Could you check a few things on this drawing? It's one solid part, dimensions in mm from its lowest x, y, z. A direction names the side the tool comes from. Coordinates: 2 decimals unless noted, no trailing zeros. Order: outer loops, then holes, each group sorted by start corner. A loop starts at its lowest first (then second) coordinate and runs counter-clockwise, first axis right, second up. Notation, with made-up numbers: (0, 53.5) -> (14, 53.5) arc R30 ccw to (14, 75.5) -> close; hole circle Ø5 at (-32, 24.25). An arc over 180 degrees is marked (long way). Use a Markdown table: item, result. Add a question column.
1. For the marked faces 1, 2 and 3, which set-ups out of +Z, -Z, +X, -X, +Y, -Y let a thin tool reach every point of the face, with its end or its side?
2. Suppose I cut it at A-A, the plane z = 8. List the corners of the cut face in (x, y) for me.
3. If I drill on line 1 along Z through (x, y) = (110, 14.5); line 2 along X through (y, z) = (2.75, 19); line 3 along X through (y, z) = (6.25, 17), over which ranges is the centre line in solid material (lowest first)? Write a range as from..to.
4. For pin 1 Ø5.5 at (y, z) = (10.5, 83.5) entering from +X; pin 2 Ø7 at (x, y) = (84.5, 11.5) entering from +Z; pin 3 Ø9 at (x, y) = (80.5, 8.5) entering from -Z, each with a flat end and sliding along its axis, tell me the tip position at first contact or that it passes through.
5. We'd pull the mould along X, two halves only. Please class the marked faces 4, 5, 6 and 7: pulls with the +X half, pulls with the -X half, needs draft (parallel to the pull), parting line crosses it, or undercut.
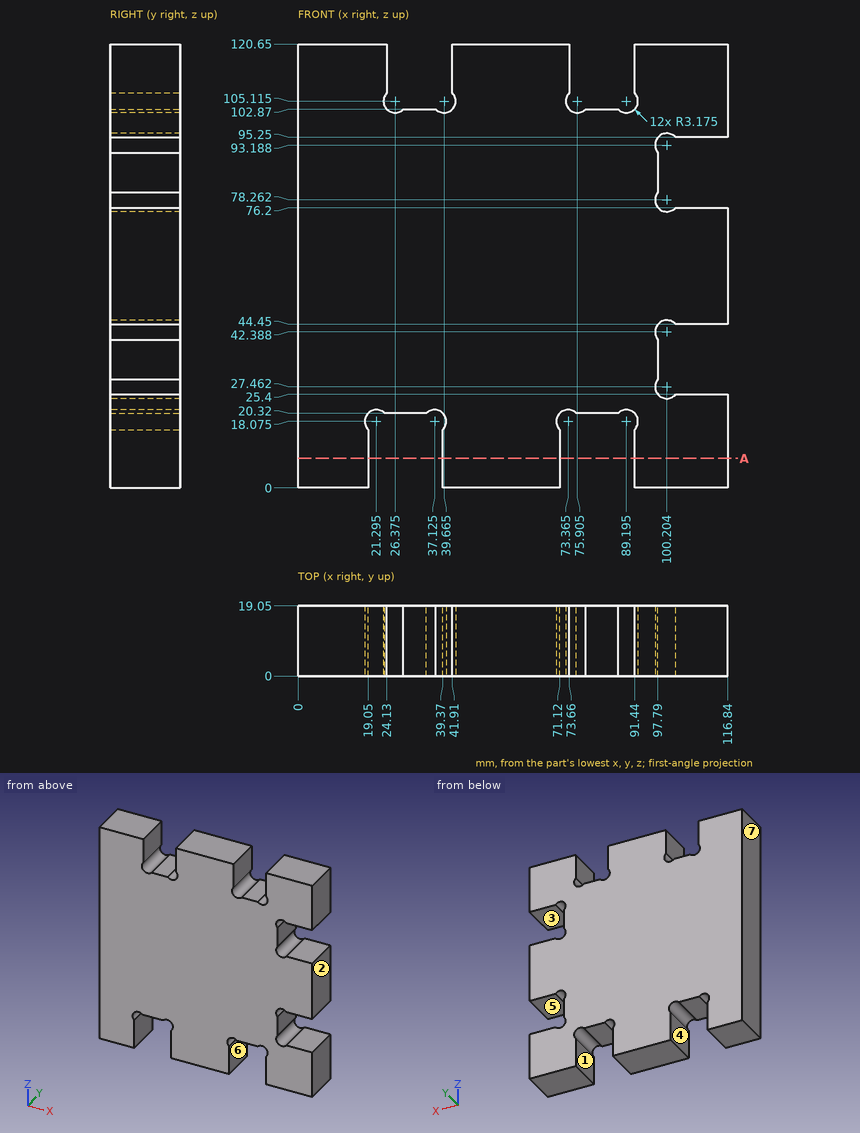
Worked out:
| question | item | result |
|---|---|---|
| 1 | face 1 | -Z, +Y, -Y |
| 1 | face 2 | +Z, -Z, +X, +Y, -Y |
| 1 | face 3 | +X, +Y, -Y |
| 2 | outline | (0, 0) -> (19.05, 0) -> (19.05, 19.05) -> (0, 19.05) -> close; (39.37, 0) -> (71.12, 0) -> (71.12, 19.05) -> (39.37, 19.05) -> close; (91.44, 0) -> (116.84, 0) -> (116.84, 19.05) -> (91.44, 19.05) -> close |
| 3 | line 1 | z = 0..25.4, 44.45..76.2, 95.25..120.65 |
| 3 | line 2 | x = 0..18.26, 40.16..70.33, 92.23..116.84 |
| 3 | line 3 | x = 0..18.31, 40.11..70.38, 92.18..116.84 |
| 4 | pin 1 | stops at x = 97.79 |
| 4 | pin 2 | stops at z = 102.87 |
| 4 | pin 3 | stops at z = 20.32 |
| 5 | face 4 | undercut |
| 5 | face 5 | needs draft |
| 5 | face 6 | undercut |
| 5 | face 7 | pulls with the -X half |
